Autodesk Inventor part; units mm, degrees
ref_plane "YZ Plane" through (0, 0, 0) normal (1, 0, 0) x (0, 1, 0)
ref_plane "XZ Plane" through (0, 0, 0) normal (0, 1, 0) x (-1, 0, 0)
ref_plane "XY Plane" through (0, 0, 0) normal (0, 0, 1) x (1, 0, 0)
sketch "草圖1" plane through (0, 0, 0) normal (0, 0, 1) x (1, 0, 0)
  circle A0 centre (0, 0) radius 60
  circle A1 centre (0, 0) radius 35
  dimension "d0" = 120
  dimension "d4" = 70
extrude "擠出1" add sketch "草圖1" along normal blind 8
sketch "草圖2" plane through (0, 0, 8) normal (0, 0, 1) x (1, 0, 0)
  circle A0 centre (0, 0) radius 60
  circle A1 centre (0, 0) radius 35
  circle A2 centre (0, 0) radius 48
  circle A3 centre (0, 0) radius 47
  dimension "d7" = 12
  dimension "d8" = 12
extrude "擠出2" cut sketch "草圖2" against normal blind 2 contours A2
sketch "草圖3" plane through (0, 0, 0) normal (0, 0, -1) x (-1, 0, 0)
  circle A0 centre (0, 0) radius 48
  circle A1 centre (0, 0) radius 47
  circle A2 centre (0, 0) radius 35
  circle A3 centre (0, 0) radius 60
extrude "擠出3" cut sketch "草圖3" against normal blind 2 contours A0
sketch "草圖4" plane through (0, 0, 8) normal (0, 0, 1) x (1, 0, 0)
  circle A0 centre (0, 0) radius 41 construction
  circle A1 centre (0, -41) radius 2.5
  circle A2 centre (0, 0) radius 41 construction
  circle A3 centre (41, 0) radius 2.5
  circle A4 centre (0, 0) radius 41 construction
  circle A5 centre (0, 41) radius 2.5
  circle A6 centre (0, 0) radius 41 construction
  circle A7 centre (-41, 0) radius 2.5
  circle A8 centre (0, 0) radius 54 construction
  circle A9 centre (0, -54) radius 2.5
  circle A10 centre (54, 0) radius 2.5
  circle A11 centre (0, 54) radius 2.5
  circle A12 centre (-54, 0) radius 2.5
  dimension "d13" = 82
  dimension "d19" = 108
  dimension "d14" = 5
  dimension "d17" = 360
  dimension "d20" = 5
  dimension "d23" = 360
extrude "擠出4" cut sketch "草圖4" against normal through all
chamfer "倒角1" distance 2.5 angle 45 4 edges at (51.5, 0, 8) (-2.5, -54, 8) (-56.5, 0, 8) (-2.5, 54, 8)
properties part number "arm bearing"
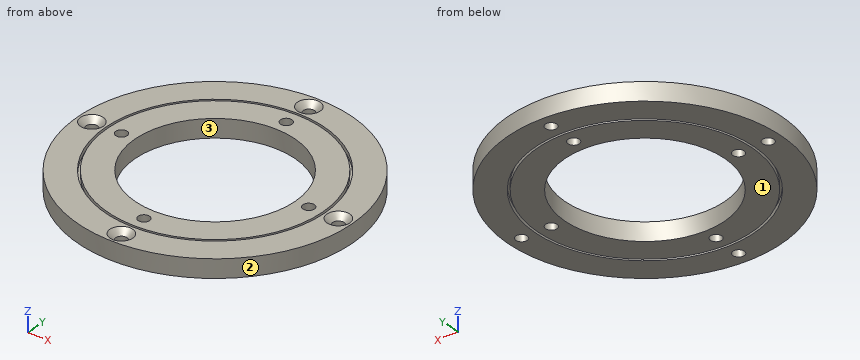
For this review, take the finished solid that the model builds, in its own axes (mm). Face numbers are marked on the shaded views. Coordinates: 2 decimals unless noted, no trailing zeros. Write each loop counter-clockwise with the first axis right and the second up, starting at its lowest first coordinate (ties: lowest second). Pieces come first, ordered by that corner, then holes. Notation, with made-up numbers: (-37.5, 42) - (15.5, 42) arc R19 ccw to (15.5, 55) - close; hole circle Ø1 at (-2.5, -12.75). An arc over 180 degrees is marked (long way). Answer in a Markdown table with one row per item. Add a question column.
Q1. We need section C-C, the plane x = -15. State the section outline as (y, z) points.
Q2. We need section A-A, the plane z = 3.25. Count the separate pieces of the cut face and the enclosed holes in it, and give its area (3 significant figures).
Q3. Draft analysis for pull direction X (two halves, no side actions). For the marked faces 1, 2 and 3, state which applies: +X half, -X half, draft (parallel to the pull), parting line (faces both ways), or undercut.
Q4. For P1, Ø1, axis at x = -12, z = 6, coming from the +Y side; P2, Ø6.5, axis at x = 0, y = 54, coming from the +Z side; P3, Ø2, axis at x = -48, z = 5, coming from the -Y side, all flat-tipped, find the tip position at first contact; note any pin that passes through.
Q5. For probe 1 along Y at (x, z) = (0, 3.75); probe 2 along X at (y, z) = (25, 0.5); probe 3 along X at (y, z) = (-14, 0.5), list the stretches that pass through material, from the lowest coordinate up.
Q6. We need section B-B, the plane y = -24. State the section outline as (x, z) points, and give its area (3 significant figures).
Answer list:
| question | item | result |
|---|---|---|
| 1 | outline | (-58.09, 0) - (-45.6, 0) - (-45.6, 2) - (-44.54, 2) - (-44.54, 0) - (-31.62, 0) - (-31.62, 8) - (-44.54, 8) - (-44.54, 6) - (-45.6, 6) - (-45.6, 8) - (-58.09, 8) - close; (31.62, 0) - (44.54, 0) - (44.54, 2) - (45.6, 2) - (45.6, 0) - (58.09, 0) - (58.09, 8) - (45.6, 8) - (45.6, 6) - (44.54, 6) - (44.54, 8) - (31.62, 8) - close |
| 2 | separate pieces | 1 |
| 2 | enclosed holes | 9 |
| 2 | area | 7,300 mm2 |
| 3 | face 1 | draft |
| 3 | face 2 | parting line |
| 3 | face 3 | undercut |
| 4 | P1 | stops at y = 58.89 |
| 4 | P2 | stops at z = 6.25 |
| 4 | P3 | stops at y = -37.3 |
| 5 | probe 1 | y = -60 to -56.5, -51.5 to -43.5, -38.5 to -35, 35 to 38.5, 43.5 to 51.5, 56.5 to 60 |
| 5 | probe 2 | x = -54.54 to -40.98, -39.8 to -24.49, 24.49 to 39.8, 40.98 to 54.54 |
| 5 | probe 3 | x = -58.34 to -45.91, -44.87 to -32.08, 32.08 to 44.87, 45.91 to 58.34 |
| 6 | outline | (-54.99, 0) - (-41.57, 0) - (-41.57, 2) - (-40.41, 2) - (-40.41, 0) - (-25.48, 0) - (-25.48, 8) - (-40.41, 8) - (-40.41, 6) - (-41.57, 6) - (-41.57, 8) - (-54.99, 8) - close; (25.48, 0) - (40.41, 0) - (40.41, 2) - (41.57, 2) - (41.57, 0) - (54.99, 0) - (54.99, 8) - (41.57, 8) - (41.57, 6) - (40.41, 6) - (40.41, 8) - (25.48, 8) - close |
| 6 | area | 463 mm2 |
